from build123d import *

# Parameters (mm, degrees)
BOSS_EXTRUDE1_DEPTH = 25.4


with BuildPart() as part:
    # Sketch1 → Boss-Extrude1 (new body)
    with BuildSketch(Plane.XY):
        with BuildLine():
            Line((2220.692415066, 2956.519458786), (2207.992415066, 2956.519458786))
            Line((2207.992415066, 2956.519458786), (2207.992415066, 2971.373508056))
            add(Edge.make_bspline(
                [(2295.101715066, 2967.625549053), (2290.064424466, 2968.346081243), (2285.012310956, 2969.008222259), (2275.661688407, 2970.095859332), (2271.46891104, 2970.561992631), (2263.712580892, 2971.284066653), (2260.22175859, 2971.544191767), (2253.376045681, 2971.962739192), (2249.944376881, 2972.130760127), (2239.630606872, 2972.494910089), (2232.684433427, 2972.539406456), (2220.026077535, 2972.178011529), (2214.353563633, 2971.875813493), (2208.634622958, 2971.424716902), (2208.420612585, 2971.407836267), (2208.206537198, 2971.390747122), (2207.992415066, 2971.373508056)],
                knots=[8.102631096, 8.102631096, 8.102631096, 8.102631096, 8.693015228, 8.693015228, 9.188395438, 9.188395438, 9.581928848, 9.581928848, 9.975462257, 9.975462257, 10.762529077, 10.762529077, 11.414127093, 11.414127093, 11.414127093, 11.438510758, 11.438510758, 11.438510758, 11.438510758], degree=3))
            Line((2295.101715066, 2967.625549053), (2295.101715066, 2935.897056736))
            Line((2295.101715066, 2935.897056736), (2288.751715066, 2935.897056736))
            Line((2288.751715066, 2935.897056736), (2288.751715066, 2943.811183941))
            Line((2288.751715066, 2943.811183941), (2282.401715066, 2943.811183941))
            Line((2282.401715066, 2943.811183941), (2282.401715066, 2956.511183941))
            Line((2282.401715066, 2956.511183941), (2278.998115066, 2956.511183941))
            Line((2278.998115066, 2956.511183941), (2278.998115066, 2943.811183941))
            Line((2278.998115066, 2943.811183941), (2233.621015066, 2947.035979773))
            Line((2233.621015066, 2947.035979773), (2233.621015066, 2959.735979773))
            Line((2233.621015066, 2959.735979773), (2230.217415066, 2959.735979773))
            Line((2230.217415066, 2959.735979773), (2230.217415066, 2947.035979773))
            Line((2230.217415066, 2947.035979773), (2225.454915066, 2947.035979773))
            Line((2225.454915066, 2947.035979773), (2225.454915066, 2937.871351382))
            Line((2225.454915066, 2937.871351382), (2220.692415066, 2937.871351382))
            Line((2220.692415066, 2937.871351382), (2220.692415066, 2956.519458786))
        make_face()
    extrude(amount=BOSS_EXTRUDE1_DEPTH)


solid = part.part
Read the model definition and answer for the solid it produces. Units are mm, in the model's axes. A direction names the side the tool comes from. Give positions to 0.01 mm unless a question says otherwise; leave off trailing zeros. Write each loop counter-clockwise with the first axis right and the second up, starting at its lowest first coordinate (ties: lowest second). Pieces come first, ordered by that corner, then holes. Notation, with made-up numbers: M 18.25,51.25 L 75.25,51.25 A25 cw 75.25,64.25 Z; hole C 36.25,23.5 d6. An arc over 180 degrees is marked long. One line per item, written item: value. Start each with the question number.
(1) Flat-ended cylindrical pins translate along their axes: pin 1 Ø3 at (x, z) = (2237.5, 18) entering from +Y; pin 2 Ø1 at (x, z) = (2232.5, 12.5) entering from -Y; pin 3 Ø1 at (x, z) = (2281, 9) entering from -Y; pin 4 Ø1 at (x, y) = (2226.5, 2962) entering from -Z. Find the tip coordinate at first contact, or state that the pin passes through.
(2) Find section A-A (y = 2954). Determine the outline of the cut face in (x, z), plus the area to 3 significant figures.
(3) Find the intervals of material crossed by line 1 (X direction, y = 2953, z = 20.25); line 2 (X direction, y = 2957, z = 7.5); line 3 (X direction, y = 2943, z = 23.5), in increasing order.
(4) A tool of negligible diameter and unlimited length cuts with its end or side. For faces 1 (the flat face through (2252, 2959, 25.4)), 2 (the flat face through (2220.692, 2947, 13)), 3 (the flat face through (2278.998, 2950, 13)), from which of +Z, -Z, +X, -X, +Y, -Y can it reach the whole face along a straight path? Write none if from no direction.
Results below:
1. pin 1: stops at y = 2972.46
1. pin 2: stops at y = 2959.74
1. pin 3: stops at y = 2956.51
1. pin 4: stops at z = 0
2. outline: M 2220.69,0 L 2230.22,0 L 2230.22,25.4 L 2220.69,25.4 Z; M 2233.62,0 L 2279,0 L 2279,25.4 L 2233.62,25.4 Z; M 2282.4,0 L 2295.1,0 L 2295.1,25.4 L 2282.4,25.4 Z
2. area: 1,720 mm^2
3. line 1: x = 2220.69 to 2230.22, 2233.62 to 2279, 2282.4 to 2295.1
3. line 2: x = 2207.99 to 2230.22, 2233.62 to 2295.1
3. line 3: x = 2220.69 to 2225.45, 2288.75 to 2295.1
4. face 1: +Z, +X, -X, +Y, -Y
4. face 2: +Z, -Z, -X, -Y
4. face 3: +Z, -Z, -Y
